Verification items for this drawing (mm, ordinates from the low corner). A direction names the side the tool comes from. Give positions to 0.01 mm unless a question says otherwise; leave off trailing zeros. Loops run counter-clockwise (first coordinate to the right, second up) from the corner with the lowest first, then second, coordinate; pieces in that order, holes last. Notation, with made-up numbers: (84, 70.5) - (124, 70.5) arc R13 ccw to (124, 80.5) - close; hole circle Ø10 at (-21.75, 51.5). An arc over 180 degrees is marked (long way). Write item = value, one per line. Start each with the question number.
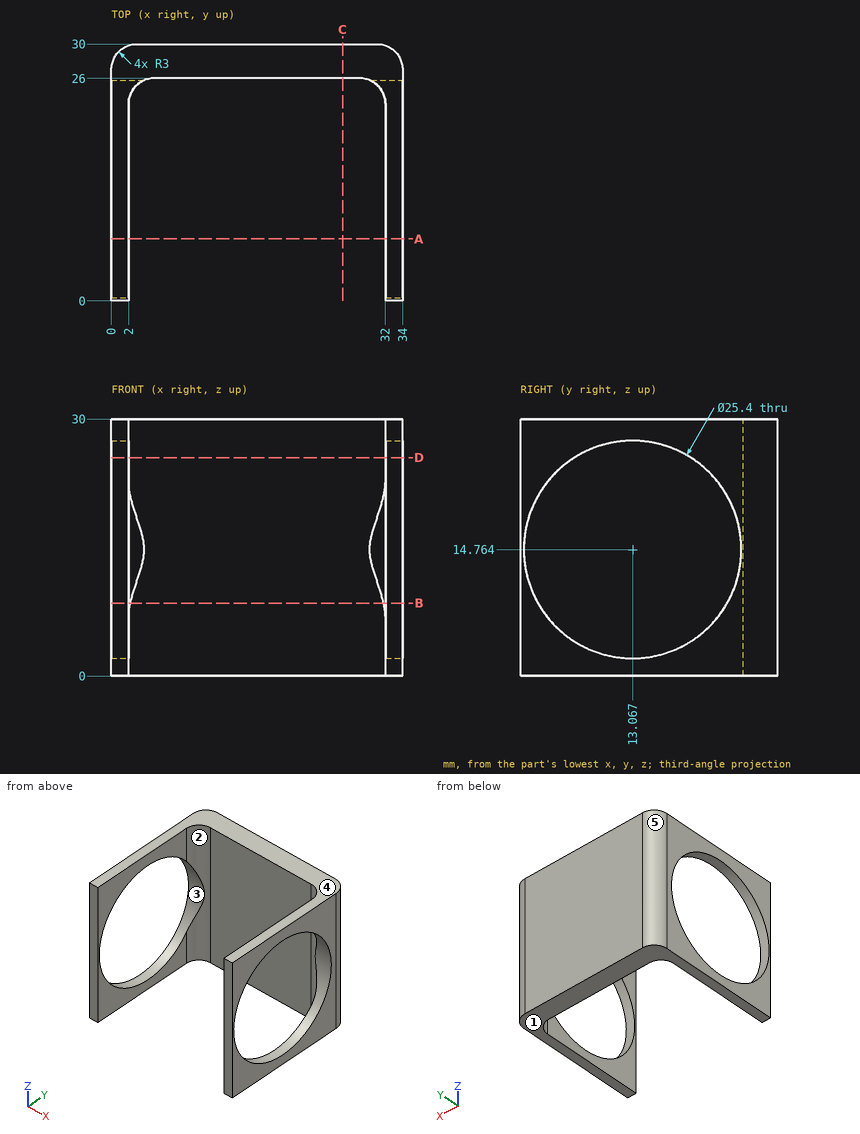
1) Cross-section at A-A on y = 7.25. Enter the section's corners in (x, z), and give its area (3 significant figures).
2) Cross-section at D-D on z = 25.5. Enter the section's corners in (x, y).
3) Cross-section at B-B on z = 8.5. Enter the section's corners in (x, y) (1 decimal), and give its area (3 significant figures).
4) Cross-section at C-C on x = 27. Enter the section's corners in (y, z).
5) Material ranges on line 1 along X through (y, z) = (5.75, 27); line 2 along Y through (x, z) = (20, 19); line 3 along X through (y, z) = (24.25, 23), recorded low to high.
6) Release check for a two-part mould opening along Z. For the marked faces 3, 4 and 5 record: pulls with the +Z half, pulls with the -Z half, needs draft (parallel to the pull), parting line crosses it, or undercut.
7) Tool access check on the marked faces 1 and 2. Record the directions out of +Z, -Z, +X, -X, +Y, -Y that give a thin tool (end or side, any length) a straight path to the whole face; none if there is none.
8) Gauge pin test, flat ends, axial feed: P1, Ø10, axis at x = 4.5, y = 19, coming from the +Z side; P2, Ø15, axis at y = 13.07, z = 14.76, coming from the -X side; P3, Ø5, axis at x = 8.5, z = 13.5, coming from the -Y side. Record the tip position at first contact, or that the pin passes through.
Checked values:
q1.outline = (0, 0) - (2, 0) - (2, 3.47) - (0, 3.47) - close; (0, 26.05) - (2, 26.05) - (2, 30) - (0, 30) - close; (32, 0) - (34, 0) - (34, 3.47) - (32, 3.47) - close; (32, 26.05) - (34, 26.05) - (34, 30) - (32, 30) - close
q1.area = 29.7 mm²
q2.outline = (0, 0) - (2, 0) - (2, 6.28) - (0, 6.28) - close; (0, 19.85) - (2, 19.85) - (2, 23) arc R3 cw to (5, 26) - (29, 26) arc R3 cw to (32, 23) - (32, 19.85) - (34, 19.85) - (34, 27) arc R3 ccw to (31, 30) - (3, 30) arc R3 ccw to (0, 27) - close; (32, 0) - (34, 0) - (34, 6.28) - (32, 6.28) - close
q3.outline = (0, 0) - (2, 0) - (2, 2) - (0, 2) - close; (0, 24.1) - (2.2, 24.1) arc R3 cw to (5, 26) - (29, 26) arc R3 cw to (31.8, 24.1) - (34, 24.1) - (34, 27) arc R3 ccw to (31, 30) - (3, 30) arc R3 ccw to (0, 27) - close; (32, 0) - (34, 0) - (34, 2) - (32, 2) - close
q3.area = 151 mm²
q4.outline = (26, 0) - (30, 0) - (30, 30) - (26, 30) - close
q5.line_1 = 0 to 2, 32 to 34
q5.line_2 = 26 to 30
q5.line_3 = 0 to 2.27, 31.73 to 34
q6.face_3 = undercut
q6.face_4 = pulls with the +Z half
q6.face_5 = needs draft
q7.face_1 = -Z, +X, -X, +Y, -Y
q7.face_2 = +Z, -Z, -Y
q8.P1 = 30
q8.P2 = through
q8.P3 = 26
